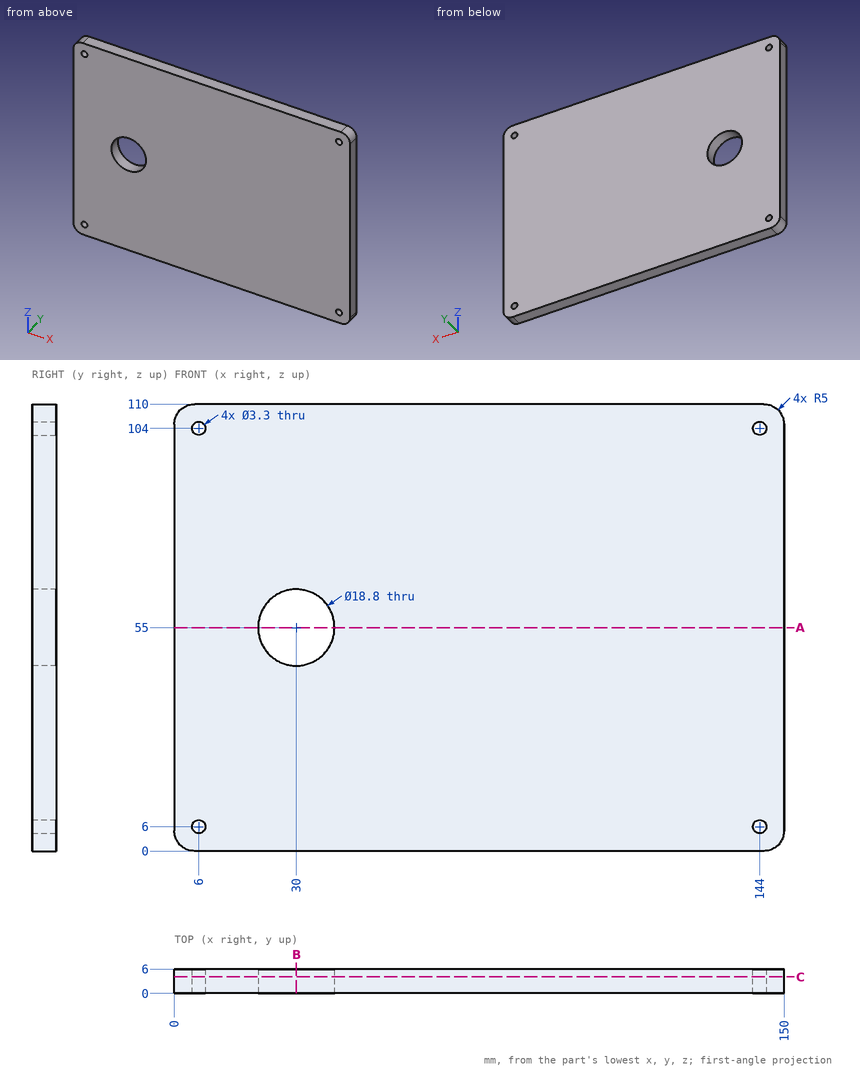
Drawing for the job (mm, zero at the part's lowest x, y, z). Give positions to 0.01 mm unless a question says otherwise; leave off trailing zeros. Order: outer loops, then holes, each group sorted by start corner. A loop starts at its lowest first (then second) coordinate and runs counter-clockwise, first axis right, second up. Notation, with made-up numbers: M 5.25,61 L 12.25,61 A36 ccw 12.25,97 Z; hole C 45.5,52 d10. An arc over 180 degrees is marked long. Put each result on its own line as item: value. Start each with the question number.
(1) Saw through at C-C, the plane y = 4.1. Write the cut outline in (x, z), then the cut area to 3 significant figures.
(2) Saw through at B-B, the plane x = 30. Write the cut outline in (y, z).
(3) Flat gauge pins, fed straight in: pin 1 Ø4.5 at (x, z) = (144, 104) entering from +Y; pin 2 Ø3 at (x, z) = (6, 104) entering from +Y. Where does each tip first touch, or does it go through?
(4) Saw through at A-A, the plane z = 55. Write the cut outline in (x, y).
(5) Drill centre lines: line 1 along Z through (x, y) = (6, 3.9); line 2 along X through (y, z) = (2.95, 104); line 3 along Z through (x, y) = (143, 1.7). Where is each one in solid material? Low to high.
Check result:
1. outline: M 0,5 A5 ccw 5,0 L 145,0 A5 ccw 150,5 L 150,105 A5 ccw 145,110 L 5,110 A5 ccw 0,105 Z; hole C 6,6 d3.3; hole C 6,104 d3.3; hole C 30,55 d18.8; hole C 144,6 d3.3; hole C 144,104 d3.3
1. area: 16,200 mm2
2. outline: M 0,0 L 6,0 L 6,45.6 L 0,45.6 Z; M 0,64.4 L 6,64.4 L 6,110 L 0,110 Z
3. pin 1: stops at y = 6
3. pin 2: passes through
4. outline: M 0,0 L 20.6,0 L 20.6,6 L 0,6 Z; M 39.4,0 L 150,0 L 150,6 L 39.4,6 Z
5. line 1: z = 0 to 4.35, 7.65 to 102.35, 105.65 to 110
5. line 2: x = 0 to 4.35, 7.65 to 142.35, 145.65 to 150
5. line 3: z = 0 to 4.69, 7.31 to 102.69, 105.31 to 110
